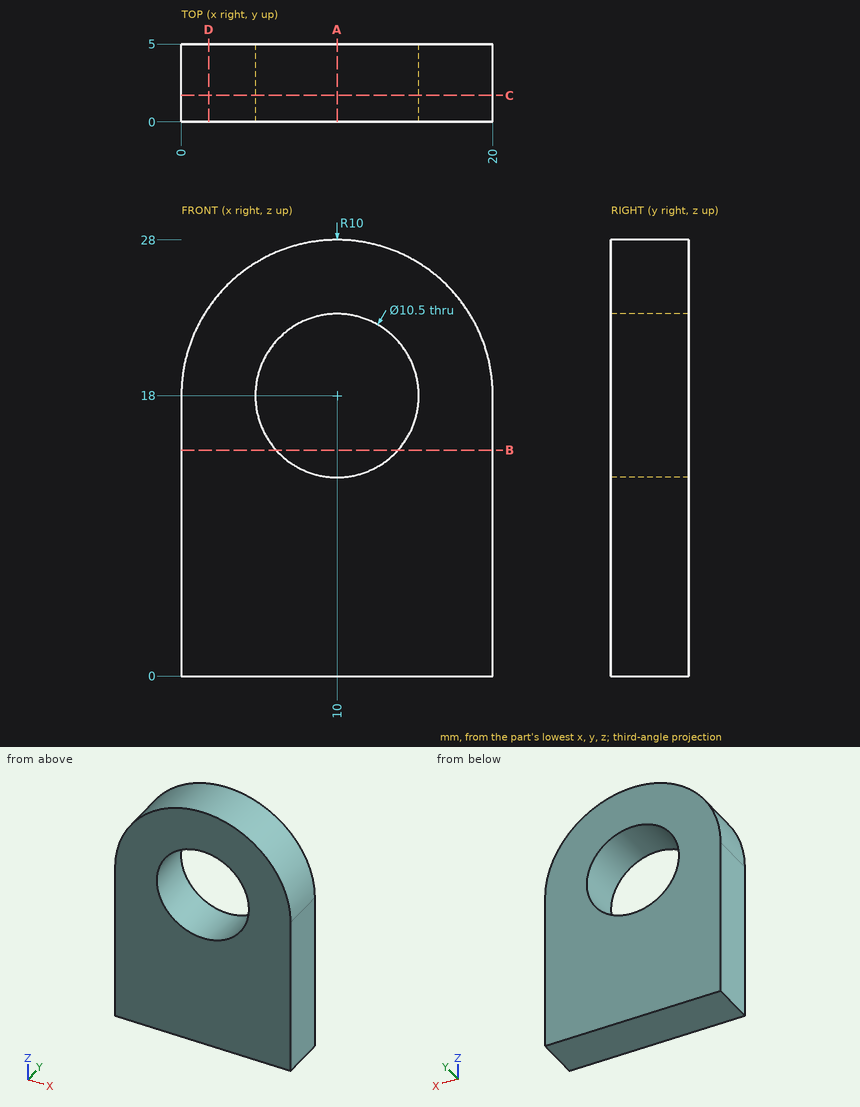
Job drawing, mm, ordinate dimensions from the low corner. One solid piece. Round coordinates to 2 decimals unless told otherwise and drop trailing zeros. Loops run counter-clockwise (first coordinate to the right, second up) from the corner with the lowest first, then second, coordinate; pieces in that order, holes last. Notation, with made-up numbers: (54.5, 21.25) -> (79.5, 21.25) arc R14 cw to (79.5, 32.25) -> close; hole circle Ø9 at (87.5, 26). An arc over 180 degrees is marked (long way). One line per item, written item: value. Start each with the question number.
Q1. Cut at B-B on z = 14.5. List the corners of the cut face in (x, y), plus the area to 3 significant figures.
Q2. Cut at D-D on x = 1.75. List the corners of the cut face in (y, z), plus the area to 3 significant figures.
Q3. Cut at C-C on y = 1.7. List the corners of the cut face in (x, z).
Q4. Cut at A-A on x = 10. List the corners of the cut face in (y, z).
Q5. Probe line 1 along Z through (x, y) = (10, 2.9); line 2 along Z through (x, y) = (12, 0.4); line 3 along X through (y, z) = (1.4, 20.5). List the from-to ranges inside material, lowest first.
Computed:
1. outline: (0, 0) -> (6.09, 0) -> (6.09, 5) -> (0, 5) -> close; (13.91, 0) -> (20, 0) -> (20, 5) -> (13.91, 5) -> close
1. area: 60.9 mm²
2. outline: (0, 0) -> (5, 0) -> (5, 23.65) -> (0, 23.65) -> close
2. area: 118 mm²
3. outline: (0, 0) -> (20, 0) -> (20, 18) arc R10 ccw to (0, 18) -> close; hole circle Ø10.5 at (10, 18)
4. outline: (0, 0) -> (5, 0) -> (5, 12.75) -> (0, 12.75) -> close; (0, 23.25) -> (5, 23.25) -> (5, 28) -> (0, 28) -> close
5. line 1: 0 to 12.75, 23.25 to 28
5. line 2: 0 to 13.15, 22.85 to 27.8
5. line 3: 0.32 to 5.38, 14.62 to 19.68
